Verification items for the finished model (mm, model axes). Face numbers are marked on the shaded views. A direction names the side the tool comes from. Coordinates: 2 decimals unless noted, no trailing zeros. Write each loop counter-clockwise with the first axis right and the second up, starting at its lowest first coordinate (ties: lowest second). Pieces come first, ordered by that corner, then holes. Notation, with made-up numbers: (-22, -28.5) - (-2, -28.5) arc R17 cw to (-2, -19.5) - close; hole circle Ø2 at (-31, 51.25). An arc over 180 degrees is marked (long way). Answer as CSV lines item,"result". Start each with the question number.
```python
from build123d import *

# Parameters (mm, degrees)
F1_DEPTH    = 25.4
F2_T1_DEPTH = 176.9830394525
F2_T3_DEPTH = 176.9830394525
F2_T5_DEPTH = 176.9830394525
F2_T7_DEPTH = 176.9830394525
F2_T9_DEPTH = 176.9830394525


# Not quite as in the source:
# - a fillet or chamfer that OpenCascade refuses, or shapes differently, is made with other operations: its cross-section is extruded or revolved along the edge and cut away or added


with BuildPart() as f1:
    # F0 (on Front) → F1 (new body)
    with BuildSketch(Plane.XZ):
        Polygon((7.0658522586, 57.8397729191), (-38.2956332455, 57.8397729191), (-60.9763759976, 18.5555741191), (-38.2956332455, -20.7286246809), (7.0658522586, -20.7286246809), (29.7465950107, 18.5555741191), align=None)
        Polygon((16.548367857, 18.5555741191), (0.4667386818, -9.2986246809), (-31.6965196687, -9.2986246809), (-47.7781488439, 18.5555741191), (-31.6965196687, 46.4097729191), (0.4667386818, 46.4097729191), align=None, mode=Mode.SUBTRACT)
    extrude(amount=-F1_DEPTH)

    # F2: chamfer of 25.4 x 11.8442145171 on 6 edges, made by hand

    # F2_s2 → F2_t1 (cut)
    with BuildSketch(Plane.YZ.offset(-104.1064102197)):
        Polygon((0, 57.8397729191), (25.4, 45.995558402), (25.4, 57.8397729191), align=None)
        Polygon((0, -20.7286246809), (25.4, -8.8844101638), (25.4, -20.7286246809), align=None)
    extrude(amount=F2_T1_DEPTH, mode=Mode.SUBTRACT)

    # F2_s4 → F2_t3 (cut)
    with BuildSketch(Plane(origin=(48.3768365242, 0, 83.7911387694), x_dir=(0, 1, 0), z_dir=(-0.5, 0, -0.8660254038))):
        Polygon((0, -62.0848777042), (25.4, -50.2406631871), (25.4, -62.0848777042), align=None)
    extrude(amount=F2_T3_DEPTH, mode=Mode.SUBTRACT)

    # F2_s6 → F2_t5 (cut)
    with BuildSketch(Plane(origin=(32.3072379553, 0, -55.9577775908), x_dir=(0, 1, 0), z_dir=(-0.5, 0, 0.8660254038))):
        Polygon((0, -35.0390940149), (25.4, -23.1948794978), (25.4, -35.0390940149), align=None)
    extrude(amount=F2_T5_DEPTH, mode=Mode.SUBTRACT)

    # F2_s8 → F2_t7 (cut)
    with BuildSketch(Plane(origin=(-40.114683202, 0, -69.4806694354), x_dir=(0, 1, 0), z_dir=(0.5, 0, 0.8660254038))):
        Polygon((0, -16.4835198958), (25.4, -4.6393053787), (25.4, -16.4835198958), align=None)
    extrude(amount=F2_T7_DEPTH, mode=Mode.SUBTRACT)

    # F2_s10 → F2_t9 (cut)
    with BuildSketch(Plane(origin=(-56.184281771, 0, 97.3140306141), x_dir=(0, 1, 0), z_dir=(0.5, 0, -0.8660254038))):
        Polygon((0, -43.5293035851), (25.4, -31.685089068), (25.4, -43.5293035851), align=None)
    extrude(amount=F2_T9_DEPTH, mode=Mode.SUBTRACT)


solid = f1.part
```
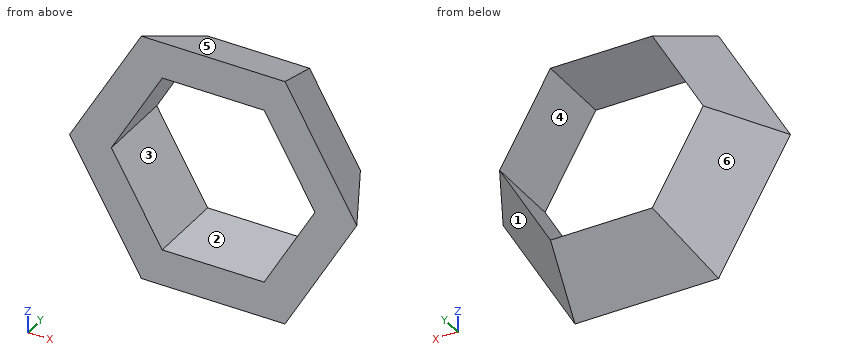
1. Draft check along X on the marked faces 3, 4, 5 and 6. Enter one of: pulls with the +X half, pulls with the -X half, needs draft (parallel to the pull), parting line crosses it, or undercut.
2. Cross-section at D-D (y = 16.5). Record the cut outline in (x, z).
3. Cross-section at C-C (z = 36). Record the cut outline in (x, y), and give its area (3 significant figures).
4. Cross-section at B-B (x = -1). Record the cut outline in (y, z).
5. Access from +Z, -Z, +X, -X, +Y, -Y to the whole of each face (thin tool, end or side, straight path). Record for the marked faces 1 and 2.
6. Depth check by flat-ended pin: P1, Ø3, axis at y = 14.5, z = 26.5, coming from the +X side; P2, Ø10, axis at x = 12, y = 13.5, coming from the +Z side; P3, Ø8, axis at x = -41, z = 42, coming from the +Y side. Enter the tip coordinate at first touch or a pass-through.
7. Cross-section at A-A (y = 5.25). Record the cut outline in (x, z), and give its area (3 significant figures).
8. Scan lines: line 1 along X through (y, z) = (23.75, 34.5); line 2 along Z through (x, y) = (-45, 23.25); line 3 along X through (y, z) = (17.5, 41.5). Record each from-to range of solid material in increasing order. Write a range as from..to.
Completed:
1,face 3,"undercut"
1,face 4,"undercut"
1,face 5,"needs draft"
1,face 6,"pulls with the -X half"
2,outline,"(-52.09, 18.56) - (-33.85, -13.03) - (2.62, -13.03) - (20.86, 18.56) - (2.62, 50.15) - (-33.85, 50.15) - close; hole (-47.78, 18.56) - (-31.7, -9.3) - (0.47, -9.3) - (16.55, 18.56) - (0.47, 46.41) - (-31.7, 46.41) - close"
3,outline,"(-50.9, 0) - (-37.71, 0) - (-37.71, 24.51) - close; (6.48, 0) - (19.68, 0) - (6.48, 24.51) - close"
3,area,"324 mm2"
4,outline,"(0, -20.73) - (24.51, -9.3) - (0, -9.3) - close; (0, 46.41) - (24.51, 46.41) - (0, 57.84) - close"
5,face 1,"-Z, +X, +Y"
5,face 2,"+Y, -Y"
6,P1,"stops at x = 18.54"
6,P2,"stops at z = 46.54"
6,P3,"stops at y = 20.54"
7,outline,"(-58.15, 18.56) - (-36.88, -18.28) - (5.65, -18.28) - (26.92, 18.56) - (5.65, 55.39) - (-36.88, 55.39) - close; hole (-47.78, 18.56) - (-31.7, -9.3) - (0.47, -9.3) - (16.55, 18.56) - (0.47, 46.41) - (-31.7, 46.41) - close"
7,area,"2,010 mm2"
8,line 1,"x = -38.98..-38.57, 7.34..7.75"
8,line 2,"z = 12.57..13.74, 23.37..24.54"
8,line 3,"x = -38.31..-34.53, 3.3..7.08"
